Source: CAD feature listing. Evaluate the final solid. Frame: model axes, mm. A direction names the side the tool comes from. Round coordinates to 2 decimals unless told otherwise and drop trailing zeros.
from build123d import *

# Parameters (mm, degrees)
SKETCH1_R           = 2.9
BOSS_EXTRUDE1_DEPTH = 4
BOSS_EXTRUDE2_DEPTH = 26.012432
SKETCH3_R           = 1.75
CUT_EXTRUDE1_DEPTH  = 79.761768867
BOSS_EXTRUDE5_DEPTH = 8.258541
CUT_EXTRUDE2_DEPTH  = 78.706037614
SKETCH6_R           = 3
CUT_EXTRUDE3_DEPTH  = 10


with BuildPart() as part:
    # Sketch1 → Boss-Extrude1 (new body)
    with BuildSketch(Plane.XY):
        with BuildLine():
            Line((-14.153385189, -69.716871134), (-10.039841479, -70.438427685))
            Line((-10.039841479, -70.438427685), (-10.231600818, -28.548135162))
            add(Edge.make_bspline(
                [(3.150526507, -12), (1.121426745, -15.448537633), (-2.522354698, -21.641292501), (-7.864373324, -26.42729642), (-10.231600818, -28.548135162)],
                knots=[0, 0, 0, 0, 0.556866484, 1, 1, 1, 1], degree=3))
            ThreePointArc((3.150526507, -12), (-3.18362895, -3.611112101), (-12.986183722, -7.406488955))
            add(Edge.make_bspline(
                [(-16.663916234, -14.630806425), (-16.157795835, -10.23676377), (-12.986183722, -7.406488955)],
                knots=[0, 0, 0, 1, 1, 1], degree=2))
            add(Edge.make_bspline(
                [(-16.663916234, -14.630806425), (-17.667702323, -19.881251045), (-18.220131563, -25.189037493), (-18.401311599, -30.514562532)],
                knots=[0, 0, 0, 0, 0.288118642, 0.288118642, 0.288118642, 0.288118642], degree=3))
            add(Edge.make_bspline(
                [(-18.401311599, -30.514562532), (-18.848969857, -43.672829442), (-17.03022033, -56.93938717), (-14.153385189, -69.716871134)],
                knots=[0.288118642, 0.288118642, 0.288118642, 0.288118642, 1, 1, 1, 1], degree=3))
        make_face()
        with Locations((-5.571628032, -12)):
            Circle(SKETCH1_R, mode=Mode.SUBTRACT)
    extrude(amount=-BOSS_EXTRUDE1_DEPTH)

    # Sketch2 → Boss-Extrude2 (add)
    with BuildSketch(Plane(origin=(0, 0, -4), x_dir=(-1, 0, 0), z_dir=(0, 0, -1))):
        with BuildLine():
            Line((10.207939206, -33.717071631), (18.466393507, -33.754875992))
            add(Edge.make_bspline(
                [(14.153385189, -69.716871134), (16.794208846, -57.987633874), (18.543433317, -45.846277061), (18.466393507, -33.754875992)],
                knots=[0.288118642, 0.288118642, 0.288118642, 0.288118642, 0.941598261, 0.941598261, 0.941598261, 0.941598261], degree=3))
            Line((14.153385189, -69.716871134), (10.039841479, -70.438427685))
            Line((10.039841479, -70.438427685), (10.207939206, -33.717071631))
        make_face()
    extrude(amount=BOSS_EXTRUDE2_DEPTH)

    # Sketch3 → Cut-Extrude1 (cut, through all)
    with BuildSketch(Plane.XY):
        with Locations((-14.103208948, -43.496863521)):
            Circle(SKETCH3_R)
        with Locations((-13.466819568, -57.346536005)):
            Circle(SKETCH3_R)
    extrude(amount=-CUT_EXTRUDE1_DEPTH, mode=Mode.SUBTRACT)

    # Sketch4 → Boss-Extrude5 (add)
    with BuildSketch(Plane(origin=(-10.362067217, -0.047433977, 0), x_dir=(0, 0, -1), z_dir=(0.9999895226985053, 0.004577607804942551, 0))):
        with BuildLine():
            Line((4, -27.831413473), (2.736644913, -37.390501041))
            Line((2.736644913, -37.390501041), (12.284980679, -33.669990424))
            add(Edge.make_bspline(
                [(4, -27.831413473), (7.157671382, -32.153592381), (12.284980679, -33.669990424)],
                knots=[0, 0, 0, 1, 1, 1], degree=2))
        make_face()
    extrude(amount=-BOSS_EXTRUDE5_DEPTH)

    # Sketch5 → Cut-Extrude2 (cut, through all)
    with BuildSketch(Plane(origin=(-10.362067217, -0.047433977, 0), x_dir=(0, 0, -1), z_dir=(0.9999895226985053, 0.004577607804942551, 0))):
        with BuildLine():
            Line((4.737663573, -38.538106349), (4.737663573, -70.391731224))
            Line((4.737663573, -70.391731224), (0, -70.391731224))
            Line((0, -70.391731224), (0, -33.715344655))
            add(Edge.make_bspline(
                [(0, -33.715344655), (4.079743683, -34.458317421), (4.737663573, -38.538106349)],
                knots=[0, 0, 0, 1, 1, 1], degree=2))
        make_face()
    extrude(amount=-CUT_EXTRUDE2_DEPTH, mode=Mode.SUBTRACT)

    # Sketch6 → Cut-Extrude3 (cut)
    with BuildSketch(Plane.XY.offset(-4.737663573)):
        with Locations((-13.466819568, -57.346536005)):
            Circle(SKETCH6_R)
        with Locations((-14.103208948, -43.496863521)):
            Circle(SKETCH6_R)
    extrude(amount=-CUT_EXTRUDE3_DEPTH, mode=Mode.SUBTRACT)


solid = part.part
1) Contact query for flat-ended pins moving along their axis: P1, Ø1, axis at y = -39.5, z = -6, coming from the -X side; P2, Ø8, axis at y = -30, z = -26.5, coming from the +X side; P3, Ø2.5, axis at x = -12.5, y = -56.5, coming from the +Z side. Output: stop coordinate, or through.
Taken from the geometry:
P1: stops at x = -18.39
P2: stops at x = -10.21
P3: stops at z = -14.74
2) Reachability of faces 4 (the face through (-14.1, -45.5, -14.738)), 5 (the face through (-13.69, -55.61, -22.27)), 6 (the face through (-13, -54, -4.738)) from +Z, -Z, +X, -X, +Y, -Y: full face, straight path, thin tool, end or side. Return the list, or none.
Taken from the geometry:
face 4: +Z
face 5: +Z, -Z
face 6: +Z, +X, -X, -Y
3) Section query A-A on z = -10. State how many separate pieces and enclosed holes the cut face has, then the cut area to 3 significant figures.
Taken from the geometry:
separate pieces: 1
enclosed holes: 2
area: 199 mm2
4) Pull-direction query (Y, two-part tool) for faces 1 (the face through (-12.13, -70.07, -17.2)), 2 (the face through (-12, -59, -14.738)), 3 (the face through (-10, -16, -4)); classes: released by +Y, released by -Y, zero draft, split by the parting line, or undercut.
Taken from the geometry:
face 1: released by -Y
face 2: undercut
face 3: zero draft
5) Material intervals for line 1 (Y direction, x = -12, z = -13.5); line 2 (Z direction, x = -2.25, y = -9); line 3 (X direction, y = -37.5, z = -19), sorted ascending.
Taken from the geometry:
line 1: y = -70.09 to -59.96, -54.73 to -45.64, -41.36 to -33.73
line 2: z = -4 to 0
line 3: x = -18.43 to -10.19
